Part model, mm, in its own coordinate system. A direction names the side the tool comes from. Round coordinates to 2 decimals unless told otherwise and drop trailing zeros. Write each loop counter-clockwise with the first axis right and the second up, starting at its lowest first coordinate (ties: lowest second). Pieces come first, ordered by that corner, then holes. Notation, with made-up numbers: (64, -1.5) -> (114, -1.5) arc R31 ccw to (114, 31.5) -> close; hole circle Ø3 at (-34.5, 71.5). An arc over 180 degrees is marked (long way). Return JSON: item names as keys, results as strings. Group by question number.
(1) Saw through at C-C (y = 58.5). List the corners of the cut face in (x, z), plus the area to 3 significant figures.
(2) Saw through at B-B (z = 2). List the corners of the cut face in (x, y).
(3) Tool access for faces 1 (the cylindrical face through (7.6, 51.275, 0.57)), 2 (the cylindrical face through (0, -8, 5)), 3 (the flat face through (0, 41, -4.5)): list every direction of +Z, -Z, +X, -X, +Y, -Y with a clear straight run to the whole face (end or side of a thin tool).
(4) Saw through at A-A (y = 36). List the corners of the cut face in (x, z).
(5) Drill centre lines: L1, parallel to Z at x = 4.5, y = -4; L2, parallel to X at y = 38.5, z = 3; L3, parallel to X at y = 1, z = 3.5. Where is each one in solid material? Low to high. Write a range as from..to.
(6) Drop flat-ended pins along their axis: pin 1 Ø5 at (y, z) = (19.5, -1.5) entering from +X; pin 2 Ø0.8 at (y, z) = (64, 5) entering from +X; pin 3 Ø0.5 at (x, z) = (1.5, 5) entering from -Y. Give the stop position or say it passes through.
(7) Mould opens along X. For faces 4 (the cylindrical face through (-1.3, 49.62, 5.01)), 5 (the cylindrical face through (0, -9, 1)), 6 (the cylindrical face through (-3.77, -2.89, -0.06)), 7 (the flat face through (-0.815, 66.94, 0.57)) say: +X half, -X half, draft (parallel to the pull), parting line (faces both ways), or undercut.
from build123d import *

# Parameters (mm, degrees)
SKETCH2_R           = 4.75
BOSS_EXTRUDE2_DEPTH = 4.5
BOSS_EXTRUDE3_START = 5.5
BOSS_EXTRUDE3_DEPTH = 10


with BuildPart() as part:
    # Sketch2 → Boss-Extrude2 (new, symmetric)
    with BuildSketch(Plane(origin=(0, 0, 0), x_dir=(0, 1, 0), z_dir=(0, 0, 1))):
        with BuildLine():
            Line((0, 8), (88, 8))
            ThreePointArc((88, 8), (90.121320344, 7.121320344), (91, 5))
            Line((91, 5), (91, -4.038605995))
            ThreePointArc((91, -4.038605995), (87.49610936, -8.007721199), (83.123062249, -5.023163597))
            ThreePointArc((83.123062249, -5.023163597), (81.466210794, -2.174908223), (78.555125766, -0.631114396))
            Line((78.555125766, -0.631114396), (56.055125766, 4.151408242))
            ThreePointArc((56.055125766, 4.151408242), (49.674974507, 1.389866291), (50.185796102, -5.543495472))
            ThreePointArc((50.185796102, -5.543495472), (50.387673623, -7.138452508), (49.030331222, -8))
            Line((49.030331222, -8), (0, -8))
            ThreePointArc((0, -8), (-8, 0), (0, 8))
        make_face()
        with Locations(Location((0, 0, 0), (0, 0, 270))):
            Circle(SKETCH2_R, mode=Mode.SUBTRACT)
    extrude(amount=BOSS_EXTRUDE2_DEPTH, both=True)

    # Sketch2<4> → Boss-Extrude3 (add)
    with BuildSketch(Plane(origin=(0, 0, 0), x_dir=(0, 1, 0), z_dir=(0, 0, 1)).offset(BOSS_EXTRUDE3_START)):
        with BuildLine():
            ThreePointArc((78.347214076, -1.609261996), (80.773118265, -2.895756853), (82.153827811, -5.269302997))
            ThreePointArc((82.153827811, -5.269302997), (87.6201367, -9), (92, -4.038605995))
            Line((92, -4.038605995), (92, 5))
            ThreePointArc((92, 5), (90.828427125, 7.828427125), (88, 9))
            Line((88, 9), (0, 9))
            ThreePointArc((0, 9), (-9, 0), (0, -9))
            Line((0, -9), (49.030331222, -9))
            ThreePointArc((49.030331222, -9), (51.292568558, -7.564087513), (50.956106022, -4.905825787))
            ThreePointArc((50.956106022, -4.905825787), (50.53042136, 0.871975682), (55.847214076, 3.173260641))
            Line((55.847214076, 3.173260641), (78.347214076, -1.609261996))
        make_face()
        with BuildLine():
            ThreePointArc((0, 8), (-8, 0), (0, -8))
            Line((0, -8), (49.030331222, -8))
            ThreePointArc((49.030331222, -8), (50.387673623, -7.138452508), (50.185796102, -5.543495472))
            ThreePointArc((50.185796102, -5.543495472), (49.674974507, 1.389866291), (56.055125766, 4.151408242))
            Line((56.055125766, 4.151408242), (78.555125766, -0.631114396))
            ThreePointArc((78.555125766, -0.631114396), (81.466210794, -2.174908223), (83.123062249, -5.023163597))
            ThreePointArc((83.123062249, -5.023163597), (87.49610936, -8.007721199), (91, -4.038605995))
            Line((91, -4.038605995), (91, 5))
            ThreePointArc((91, 5), (90.121320344, 7.121320344), (88, 8))
            Line((88, 8), (0, 8))
        make_face(mode=Mode.SUBTRACT)
    extrude(amount=-BOSS_EXTRUDE3_DEPTH)


solid = part.part
Computed values:
{
 "1": {"outline": "(-9, -4.5) -> (-2.61, -4.5) -> (-2.61, 5.5) -> (-3.63, 5.5) -> (-3.63, 4.5) -> (-8, 4.5) -> (-8, 5.5) -> (-9, 5.5) -> close", "area": "59.5 mm2"},
 "2": {"outline": "(-9, 0) arc R9 ccw to (9, 0) -> (9, 49.03) arc R2.5 ccw to (4.91, 50.96) arc R5 cw to (-3.17, 55.85) -> (1.61, 78.35) arc R5 cw to (5.27, 82.15) arc R5 ccw to (4.04, 92) -> (-5, 92) arc R4 ccw to (-9, 88) -> close; hole circle Ø9.5 at (0, 0)"},
 "3": {"face 1": "+Z, -Z", "face 2": "+Z", "face 3": "-Z, +X, -X, +Y, -Y"},
 "4": {"outline": "(-9, -4.5) -> (9, -4.5) -> (9, 5.5) -> (8, 5.5) -> (8, 4.5) -> (-8, 4.5) -> (-8, 5.5) -> (-9, 5.5) -> close"},
 "5": {"L1": "-4.5..4.5", "L2": "-9..9", "L3": "-9..-4.64, 4.64..9"},
 "6": {"pin 1": "x = 9", "pin 2": "x = -1.36", "pin 3": "y = -8.91"},
 "7": {"face 4": "undercut", "face 5": "parting line", "face 6": "undercut", "face 7": "+X half"}
}
